Geometry check sheet. Reference: the model listing, model coordinates, mm. Face numbers are marked on the shaded views. A direction names the side the tool comes from. Coordinates: 2 decimals unless noted, no trailing zeros. Write each loop counter-clockwise with the first axis right and the second up, starting at its lowest first coordinate (ties: lowest second). Pieces come first, ordered by that corner, then holes. Notation, with made-up numbers: (-15.75, 11) -> (31.25, 11) arc R22 cw to (31.25, 49) -> close; hole circle Ø2 at (37, 73). An arc over 180 degrees is marked (long way). Answer as CSV lines item,"result".
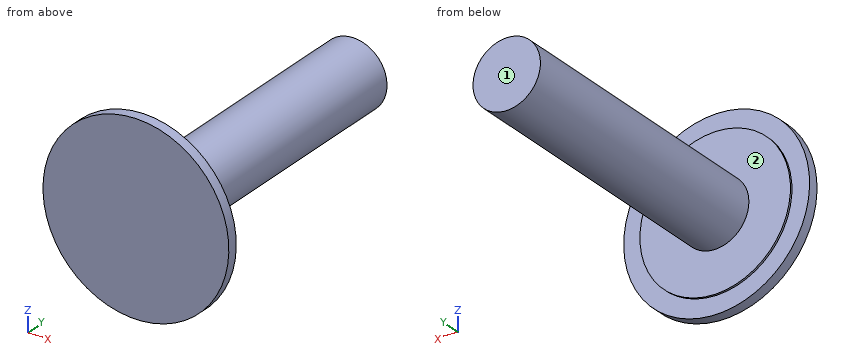
```python
from build123d import *

# Parameters (mm, degrees)
SKETCH1_R           = 11.025
BOSS_EXTRUDE1_DEPTH = 1.5
CUT_EXTRUDE1_START  = -0.25
SKETCH2_R           = 11.025
SKETCH2_R_2         = 8.930457304
CUT_EXTRUDE1_DEPTH  = 0.25
SKETCH3_R           = 4
BOSS_EXTRUDE2_DEPTH = 35


with BuildPart() as part:
    # Sketch1 → Boss-Extrude1 (new body)
    with BuildSketch(Plane(origin=(0, 0, 0), x_dir=(1, 0, 0), z_dir=(0, 1, 0))):
        with Locations(Location((0, 0, 0), (0, 0, 270))):
            Circle(SKETCH1_R)
    extrude(amount=BOSS_EXTRUDE1_DEPTH)

    # Sketch2 → Cut-Extrude1 (cut)
    with BuildSketch(Plane(origin=(0, 1.5, 0), x_dir=(1, 0, 0), z_dir=(0, 1, 0)).offset(CUT_EXTRUDE1_START)):
        with Locations(Location((0, 0, 0), (0, 0, 270))):
            Circle(SKETCH2_R)
        with Locations(Location((0, 0, 0), (0, 0, 270))):
            Circle(SKETCH2_R_2, mode=Mode.SUBTRACT)
    extrude(amount=CUT_EXTRUDE1_DEPTH, mode=Mode.SUBTRACT)

    # Sketch3 → Boss-Extrude2 (add)
    with BuildSketch(Plane(origin=(0, 1.5, 0), x_dir=(1, 0, 0), z_dir=(0, 1, 0))):
        with Locations(Location((0, 0, 0), (0, 0, 270))):
            Circle(SKETCH3_R)
    extrude(amount=BOSS_EXTRUDE2_DEPTH)


solid = part.part
```
Item 1: Cross-section at A-A, the plane z = 0. Record the cut outline in (x, y) (3 decimals), plus the area to 3 significant figures.
Responses:
outline,"(-11.025, 0) -> (11.025, 0) -> (11.025, 1.25) -> (8.93, 1.25) -> (8.93, 1.5) -> (4, 1.5) -> (4, 36.5) -> (-4, 36.5) -> (-4, 1.5) -> (-8.93, 1.5) -> (-8.93, 1.25) -> (-11.025, 1.25) -> close"
area,"312 mm2"
Item 2: Depth check by flat-ended pin: pin 1 Ø2 at (x, y) = (-1, 20.5) entering from +Z; pin 2 Ø3 at (x, z) = (7, -8) entering from +Y; pin 3 Ø5 at (x, y) = (4, 16) entering from +Z. Enter the tip coordinate at first touch or a pass-through.
Responses:
pin 1,"stops at z = 4"
pin 2,"stops at y = 1.25"
pin 3,"stops at z = 3.71"
Item 3: Thickness scan on probe 1 along Y at (x, z) = (-5.75, -1); probe 2 along X at (y, z) = (22, 0.25); probe 3 along X at (y, z) = (14.5, -1.5). Record the ranges inside material, lowest first.
Responses:
probe 1,"y = 0 to 1.5"
probe 2,"x = -3.99 to 3.99"
probe 3,"x = -3.71 to 3.71"
Item 4: Cross-section at D-D, the plane z = 7. Record the cut outline in (x, y), plus the area to 3 significant figures.
Responses:
outline,"(-8.52, 0) -> (8.52, 0) -> (8.52, 1.25) -> (5.55, 1.25) -> (5.55, 1.5) -> (-5.55, 1.5) -> (-5.55, 1.25) -> (-8.52, 1.25) -> close"
area,"24.1 mm2"
Item 5: Cross-section at C-C, the plane y = 17. Record the cut outline in (x, z).
Responses:
outline,"circle Ø8 at (0, 0)"
Item 6: Set-up check for the marked faces 1 and 2: record each of +Z, -Z, +X, -X, +Y, -Y from which the full face is reachable in a straight line by a thin tool's end or side.
Responses:
face 1,"+Z, -Z, +X, -X, +Y"
face 2,"+Y"
Item 7: Cross-section at B-B, the plane x = 0. Record the cut outline in (y, z) (3 decimals).
Responses:
outline,"(0, -11.025) -> (1.25, -11.025) -> (1.25, -8.93) -> (1.5, -8.93) -> (1.5, -4) -> (36.5, -4) -> (36.5, 4) -> (1.5, 4) -> (1.5, 8.93) -> (1.25, 8.93) -> (1.25, 11.025) -> (0, 11.025) -> close"
